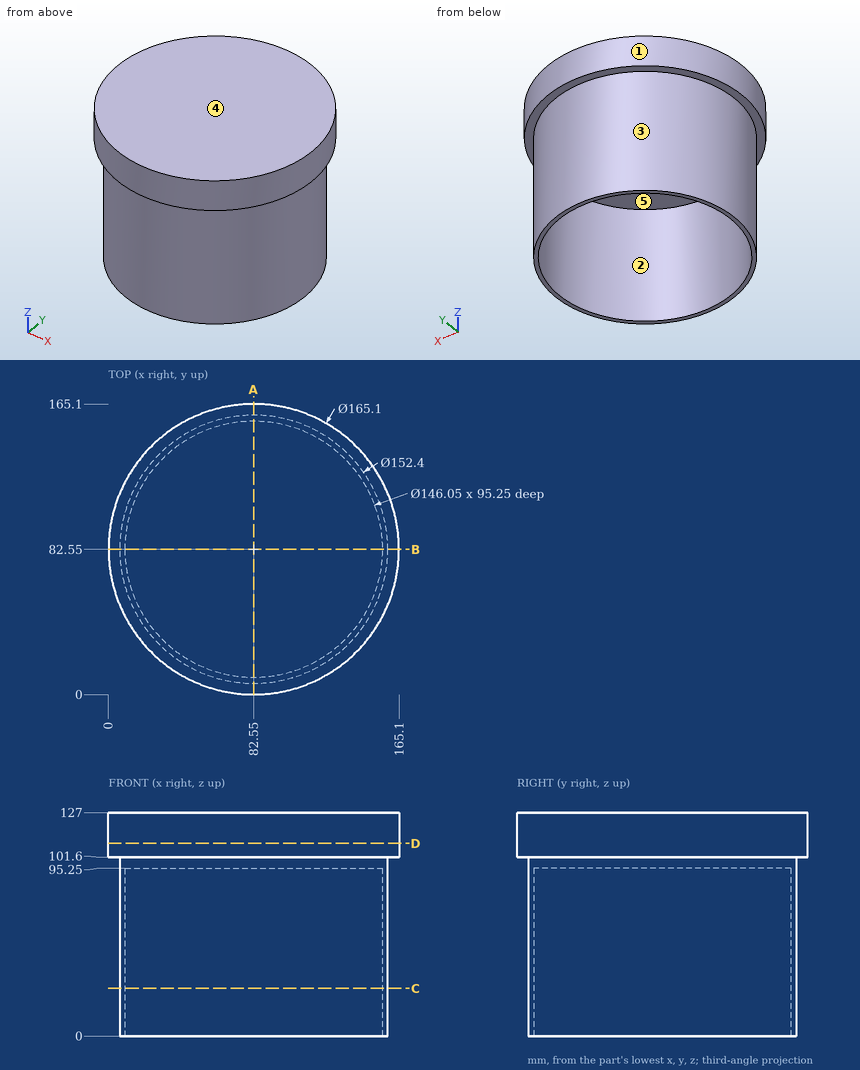
The drawing under review shows one solid part. Ordinate dimensions are in mm from its lowest x, y, z. A direction names the side the tool comes from. Round coordinates to 2 decimals unless told otherwise and drop trailing zeros. Loops run counter-clockwise (first coordinate to the right, second up) from the corner with the lowest first, then second, coordinate; pieces in that order, holes last.
Item 1: Take a section at D-D (z = 109.5). Write out the cut boundary in (x, y), then the cut area to 3 significant figures.
Determined:
outline: circle Ø165.1 at (82.55, 82.55)
area: 21,400 mm2
Item 2: Take a section at C-C (z = 27). Write out the cut boundary in (x, y) (3 decimals).
Determined:
outline: circle Ø152.4 at (82.55, 82.55); hole circle Ø146.05 at (82.55, 82.55)
Item 3: For the marked faces 1 and 2, list the 3-axis set-ups (+Z, -Z, +X, -X, +Y, -Y) from which the entire face can be reached by the end or side of a thin tool; tool diameter is ignored.
Determined:
face 1: +Z, -Z
face 2: -Z
Item 4: Take a section at A-A (x = 82.55). Write out the cut boundary in (y, z) (3 decimals), then the cut area to 3 significant figures.
Determined:
outline: (0, 101.6) - (6.35, 101.6) - (6.35, 0) - (9.525, 0) - (9.525, 95.25) - (155.575, 95.25) - (155.575, 0) - (158.75, 0) - (158.75, 101.6) - (165.1, 101.6) - (165.1, 127) - (0, 127) - close
area: 5,770 mm2
Item 5: Mouldability with a two-part tool opening along Y and no side actions: class the marked faces 3, 4 and 5 as released by +Y, released by -Y, zero draft, split by the parting line, or undercut.
Determined:
face 3: split by the parting line
face 4: zero draft
face 5: undercut
Item 6: Clearance check with flat-ended pins moving along their axes: pin 1 Ø8 at (x, z) = (87.5, 41.5) entering from -Y; pin 2 Ø5 at (x, y) = (72.5, 107) entering from -Z; pin 3 Ø5 at (x, z) = (129, 81) entering from -Y. State where each tip first meets the part, or that it passes through.
Determined:
pin 1: stops at y = 6.36
pin 2: stops at z = 95.25
pin 3: stops at y = 20.3
Item 7: For line 1 (Y direction, x = 82.55, z = 33) (3 decimals); line 2 (X direction, y = 82, z = 75); line 3 (Z direction, x = 91.5, y = 70), list the stretches that pass through material, from the lowest coordinate up.
Determined:
line 1: y = 6.35 to 9.525, 155.575 to 158.75
line 2: x = 6.35 to 9.53, 155.57 to 158.75
line 3: z = 95.25 to 127
